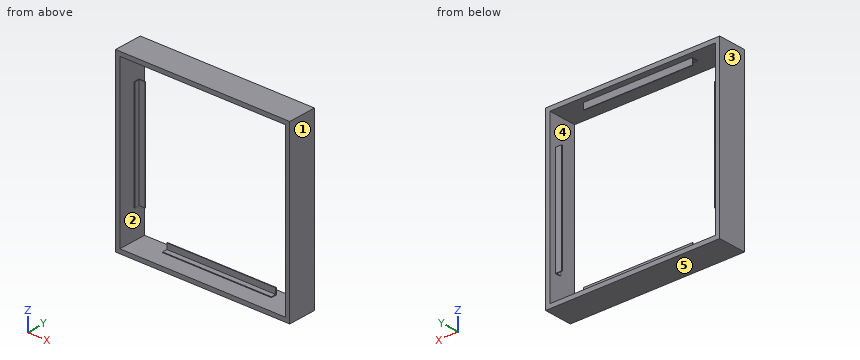
Autodesk Inventor part; units mm, degrees
ref_plane "YZ Plane" through (0, 0, 0) normal (1, 0, 0) x (0, 1, 0)
ref_plane "XZ Plane" through (0, 0, 0) normal (0, 1, 0) x (-1, 0, 0)
ref_plane "XY Plane" through (0, 0, 0) normal (0, 0, 1) x (1, 0, 0)
sketch "Sketch15" plane through (0, 0, 0) normal (0, 1, 0) x (-1, 0, 0)
  line L0 (-369.8875, -368.1356) -> (369.8875, -368.1356)
  line L1 (369.8875, -368.1356) -> (369.8875, 368.4644)
  line L2 (369.8875, 368.4644) -> (-369.8875, 368.4644)
  line L3 (-369.8875, 368.4644) -> (-369.8875, -368.1356)
  line L4 (-389.0391, -387.2872) -> (389.0391, -387.2872)
  line L5 (389.0391, -387.2872) -> (389.0391, 387.616)
  line L6 (389.0391, 387.616) -> (-389.0391, 387.616)
  line L7 (-389.0391, 387.616) -> (-389.0391, -387.2872)
  dimension "d84" = 736.6
  dimension "d85" = 739.775
  dimension "d86" = 19.1516
  dimension "d87" = 19.1516
  dimension "d88" = 19.1516
  dimension "d89" = 19.1516
extrude "Extrusion12" add sketch "Sketch15" along normal blind 127
sketch "Sketch16" plane through (-369.8875, 0, -368.1356) normal (1, 0, 0) x (0, 0, -1)
  line L0 (-609.6, 73.66) -> (-127, 73.66)
  line L1 (-127, 73.66) -> (-127, 99.06)
  line L2 (-127, 99.06) -> (-609.6, 99.06)
  line L3 (-609.6, 99.06) -> (-609.6, 73.66)
  line L4 (-736.6, 0) -> (-736.6, 127)
  line L5 (0, 0) -> (0, 127)
  line L6 (0, 0) -> (-736.6, 0)
  point P0 (-368.1356, 0)
  dimension "d92" = 127
  dimension "d93" = 127
  dimension "d94" = 73.66
  dimension "d95" = 25.4
sketch "Sketch17" plane through (-369.8875, 0, -368.1356) normal (0, 0, 1) x (1, 0, 0)
  line L0 (127, 73.66) -> (612.775, 73.66)
  line L1 (612.775, 73.66) -> (612.775, 99.06)
  line L2 (612.775, 99.06) -> (127, 99.06)
  line L3 (127, 99.06) -> (127, 73.66)
  line L4 (0, 0) -> (0, 127)
  line L5 (739.775, 0) -> (739.775, 127)
  line L6 (739.775, 0) -> (0, 0)
  point P0 (369.8875, 0)
  dimension "d96" = 127
  dimension "d97" = 127
  dimension "d98" = 25.4
  dimension "d99" = 73.66
sketch "Sketch18" plane through (369.8875, 0, 368.4644) normal (-1, 0, 0) x (0, 0, 1)
  line L0 (-609.6, 73.66) -> (-127, 73.66)
  line L1 (-127, 73.66) -> (-127, 99.06)
  line L2 (-127, 99.06) -> (-609.6, 99.06)
  line L3 (-609.6, 99.06) -> (-609.6, 73.66)
  line L4 (-736.6, 0) -> (-736.6, 127)
  line L5 (0, 0) -> (0, 127)
  line L6 (0, 0) -> (-736.6, 0)
  point P0 (-368.4644, 0)
  dimension "d100" = 127
  dimension "d101" = 127
  dimension "d102" = 25.4
  dimension "d103" = 73.66
sketch "Sketch19" plane through (369.8875, 0, 368.4644) normal (0, 0, -1) x (-1, 0, 0)
  line L0 (127, 73.66) -> (612.775, 73.66)
  line L1 (612.775, 73.66) -> (612.775, 99.06)
  line L2 (612.775, 99.06) -> (127, 99.06)
  line L3 (127, 99.06) -> (127, 73.66)
  line L4 (739.775, 0) -> (739.775, 127)
  line L5 (739.775, 0) -> (0, 0)
  point P0 (369.8875, 0)
  point P1 (0, 127)
  dimension "d104" = 127
  dimension "d105" = 127
  dimension "d106" = 25.4
  dimension "d107" = 73.66
extrude "Extrusion13" add sketch "Sketch19" along normal blind 3.175
extrude "Extrusion14" add sketch "Sketch16" along normal blind 3.175
extrude "Extrusion15" add sketch "Sketch18" along normal blind 3.175
extrude "Extrusion16" add sketch "Sketch17" along normal blind 3.175
sketch "Sketch20" plane through (-369.8875, 0, -364.9606) normal (0, 0, 1) x (1, 0, 0)
  line L0 (612.775, 99.06) -> (127, 99.06)
  line L1 (127, 99.06) -> (127, 73.66)
  line L2 (612.775, 99.06) -> (127, 99.06)
  line L3 (127, 99.06) -> (127, 95.885)
  line L4 (127, 95.885) -> (612.775, 95.885)
  line L5 (612.775, 95.885) -> (612.775, 99.06)
  point P0 (369.8875, 0)
  dimension "d116" = 3.175
extrude "Extrusion17" add sketch "Sketch20" along normal blind 25.4
sketch "Sketch21" plane through (366.7125, 0, 368.4644) normal (-1, 0, 0) x (0, 0, 1)
  line L0 (-609.6, 99.06) -> (-127, 99.06)
  line L1 (-609.6, 99.06) -> (-609.6, 73.66)
  line L2 (-127, 99.06) -> (-609.6, 99.06)
  line L3 (-609.6, 99.06) -> (-609.6, 95.885)
  line L4 (-609.6, 95.885) -> (-127, 95.885)
  line L5 (-127, 95.885) -> (-127, 99.06)
  point P0 (-368.4644, 0)
  dimension "d119" = 3.175
sketch "Sketch22" plane through (369.8875, 0, 365.2894) normal (0, 0, -1) x (-1, 0, 0)
  line L0 (612.775, 73.66) -> (612.775, 99.06)
  line L1 (127, 99.06) -> (612.775, 99.06)
  line L2 (612.775, 99.06) -> (612.775, 95.885)
  line L3 (612.775, 95.885) -> (127, 95.885)
  line L4 (127, 95.885) -> (127, 99.06)
  point P0 (369.8875, 0)
  dimension "d120" = 3.175
extrude "Extrusion18" add sketch "Sketch22" along normal blind 25.4
extrude "Extrusion19" add sketch "Sketch21" along normal blind 25.4
sketch "Sketch23" plane through (-366.7125, 0, -368.1356) normal (1, 0, 0) x (0, 0, -1)
  line L0 (-609.6, 99.06) -> (-127, 99.06)
  line L1 (-127, 99.06) -> (-127, 73.66)
  line L2 (-609.6, 99.06) -> (-127, 99.06)
  line L3 (-127, 99.06) -> (-127, 95.885)
  line L4 (-127, 95.885) -> (-609.6, 95.885)
  line L5 (-609.6, 95.885) -> (-609.6, 99.06)
  point P0 (-368.1356, 0)
  dimension "d125" = 3.175
extrude "Extrusion20" add sketch "Sketch23" along normal blind 25.4
equation "\"d87\" = d86"
equation "\"d88\" = d86"
equation "\"d89\" = d86"
equation "\"d93\" = d92"
equation "\"d96\" = d92"
equation "\"d97\" = d92"
equation "\"d100\" = d92"
equation "\"d101\" = d92"
equation "\"d105\" = d92"
equation "\"d119\" = d116"
equation "\"d120\" = d116"
equation "\"d125\" = d116"
properties part number "Bumper"
Part model, mm, in its own coordinate system. Face numbers are marked on the shaded views. A direction names the side the tool comes from. Round coordinates to 2 decimals unless told otherwise and drop trailing zeros. Write each loop counter-clockwise with the first axis right and the second up, starting at its lowest first coordinate (ties: lowest second). Pieces come first, ordered by that corner, then holes. Notation, with made-up numbers: M 65.5,61 L 70.5,61 A25 cw 70.5,96 Z; hole C 3,86.25 d3. An arc over 180 degrees is marked long. Return JSON: item names as keys, results as strings. Group by question number.
(1) Saw through at C-C on y = 24.5. Write the cut outline in (x, z), then the cut area to 3 significant figures.
(2) Pin check, flat tips, straight feed: pin 1 Ø2.5 at (x, z) = (2.5, -366) entering from -Y; pin 2 Ø7.5 at (x, z) = (-349, -109) entering from -Y (3 decimals). Stop position of each tip, or through.
(3) Saw through at B-B on x = 314. Write the cut outline in (y, z), then the cut area to 3 significant figures.
(4) Saw through at D-D on x = -216.5. Write the cut outline in (y, z) (3 decimals), then the cut area to 3 significant figures.
(5) Which spindle directions (+Z, -Z, +X, -X, +Y, -Y) get a long thin tool onto all of the face, cutting with end or side? Do the marked faces 4 and 5. Say none if no direction does.
(6) Two-plate mould, pull along X, no slides. Class the marked faces 1, 2 and 3: +X half, -X half, draft (parallel to the pull), parting line (faces both ways), or undercut.
(7) Drill centre lines: probe 1 along Z at (x, y) = (-319.5, 75); probe 2 along Z at (x, y) = (-224, 84.5); probe 3 along X at (y, z) = (42, 326). Where is each one in solid material? Low to high.
(8) Saw through at A-A on z = 269. Write the cut outline in (x, y).
Returned:
{
 "1": {"outline": "M -389.04,-387.29 L 389.04,-387.29 L 389.04,387.62 L -389.04,387.62 Z; hole M -369.89,-368.14 L 369.89,-368.14 L 369.89,368.46 L -369.89,368.46 Z", "area": "58,000 mm²"},
 "2": {"pin 1": "y = 73.66", "pin 2": "y = 95.885"},
 "3": {"outline": "M 0,-387.29 L 127,-387.29 L 127,-368.14 L 0,-368.14 Z; M 0,368.46 L 127,368.46 L 127,387.62 L 0,387.62 Z", "area": "4,860 mm²"},
 "4": {"outline": "M 0,-387.287 L 127,-387.287 L 127,-368.136 L 99.06,-368.136 L 99.06,-339.561 L 95.885,-339.561 L 95.885,-364.961 L 73.66,-364.961 L 73.66,-368.136 L 0,-368.136 Z; M 0,368.464 L 73.66,368.464 L 73.66,365.289 L 95.885,365.289 L 95.885,339.889 L 99.06,339.889 L 99.06,368.464 L 127,368.464 L 127,387.616 L 0,387.616 Z", "area": "5,190 mm²"},
 "5": {"face 4": "none", "face 5": "-Z, +X, -X, +Y, -Y"},
 "6": {"face 1": "+X half", "face 2": "undercut", "face 3": "-X half"},
 "7": {"probe 1": "-387.29 to -368.14, 368.46 to 387.62", "probe 2": "-387.29 to -364.96, 365.29 to 387.62", "probe 3": "-389.04 to -369.89, 369.89 to 389.04"},
 "8": {"outline": "M -389.04,0 L -369.89,0 L -369.89,127 L -389.04,127 Z; M 369.89,0 L 389.04,0 L 389.04,127 L 369.89,127 Z"}
}
